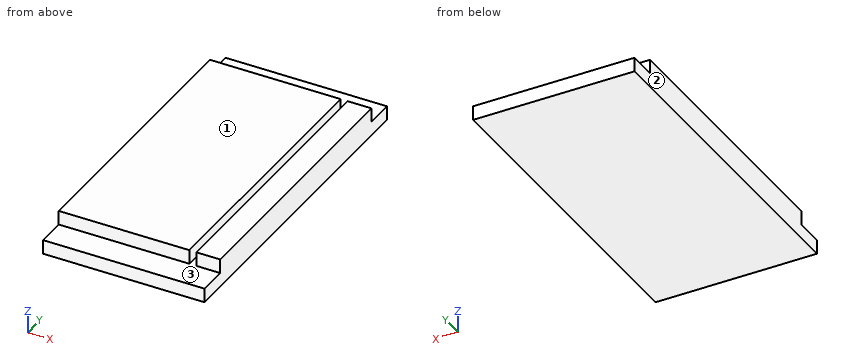
from build123d import *

# Parameters (mm, degrees)
F0_W     = 68
F0_H     = 12
F1_DEPTH = 140
F2_W     = 3
F2_H     = 6
F3_DEPTH = 140
F4_W     = 12
F4_H     = 6
F5_DEPTH = 70


with BuildPart() as f1:
    # F0 (on Front) → F1 (new body)
    with BuildSketch(Plane.XZ):
        Rectangle(F0_W, F0_H)
    extrude(amount=F1_DEPTH)

    # F2 (on face) → F3 (cut)
    with BuildSketch(Plane.XZ.offset(140)):
        with Locations((22.5, 3)):
            Rectangle(F2_W, F2_H)
    extrude(amount=-F3_DEPTH, mode=Mode.SUBTRACT)

    # F4 (on face) → F5 (cut)
    with BuildSketch(Plane(origin=(-34, 0, 0), x_dir=(0, -1, 0), z_dir=(-1, 0, 0))):
        with Locations((6, 3)):
            Rectangle(F4_W, F4_H)
        with Locations((134, 3)):
            Rectangle(F4_W, F4_H)
    extrude(amount=-F5_DEPTH, mode=Mode.SUBTRACT)


solid = f1.part
Source: CAD feature listing. Evaluate the final solid. Frame: model axes, mm. Face numbers are marked on the shaded views. Round coordinates to 2 decimals unless told otherwise and drop trailing zeros. Order: outer loops, then holes, each group sorted by start corner. A loop starts at its lowest first (then second) coordinate and runs counter-clockwise, first axis right, second up. Notation, with made-up numbers: (80.25, -24.5) - (124.25, -24.5) arc R30 cw to (124.25, 4.5) - close; hole circle Ø4 at (-4.75, 40). An arc over 180 degrees is marked (long way). Use a Markdown table: item, result. Add a question column.
1. Section query B-B (y = -31.5). Return the cut outline in (x, z), then the cut area to 3 significant figures.
2. Line query: probe 1 along X at (y, z) = (-100.5, 2.25); probe 2 along Y at (x, z) = (-1, 4.75); probe 3 along Z at (x, y) = (21.5, -25). Output: solid intervals per line, ascending.
3. Section query A-A (z = 3.75). Return the cut outline in (x, y), then the cut area to 3 significant figures.
4. Section query D-D (y = -131). Return the cut outline in (x, z), then the cut area to 3 significant figures.
5. Mould query, pull axis X, two halves, no side actions, for the marked faces 1, 2 and 3. Classes: +X half, -X half, draft (parallel to the pull), parting line (faces both ways), or undercut.
6. First-contact query: pin 1 (3 mm diameter, centred on x = 30, z = 4.5, fed in from -Y); pin 2 (1 mm diameter, centred on x = 9, z = 4, fed in from +Y). Flat tips, straight axial feed; report the tip coordinate or a pass-through.
7. Section query C-C (x = 10). Return the cut outline in (y, z).
Derived:
| question | item | result |
|---|---|---|
| 1 | outline | (-34, -6) - (34, -6) - (34, 6) - (24, 6) - (24, 0) - (21, 0) - (21, 6) - (-34, 6) - close |
| 1 | area | 798 mm2 |
| 2 | probe 1 | -34 to 21, 24 to 34 |
| 2 | probe 2 | -128 to -12 |
| 2 | probe 3 | -6 to 0 |
| 3 | outline | (-34, -128) - (21, -128) - (21, -12) - (-34, -12) - close; (24, -128) - (34, -128) - (34, -12) - (24, -12) - close |
| 3 | area | 7,540 mm2 |
| 4 | outline | (-34, -6) - (34, -6) - (34, 0) - (-34, 0) - close |
| 4 | area | 408 mm2 |
| 5 | face 1 | draft |
| 5 | face 2 | -X half |
| 5 | face 3 | undercut |
| 6 | pin 1 | y = -128 |
| 6 | pin 2 | y = -12 |
| 7 | outline | (-140, -6) - (0, -6) - (0, 0) - (-12, 0) - (-12, 6) - (-128, 6) - (-128, 0) - (-140, 0) - close |
